from build123d import *

# Parameters (mm, degrees)
F1_DEPTH = 25.4
F2_T     = -2.54


with BuildPart() as f1:
    # F0 (on Front) → F1 (new body)
    with BuildSketch(Plane.XZ):
        with BuildLine():
            ThreePointArc((-49.597935, -5.970298), (-42.262804, 19.828677), (-16.245349, 26.3466))
            ThreePointArc((-16.245349, 26.3466), (-60.981474, 39.147241), (-49.597935, -5.970298))
        make_face()
        with BuildLine():
            ThreePointArc((-49.597935, -5.970298), (-26.099746, -1.543581), (-15.451481, 19.866116))
            ThreePointArc((-15.451481, 19.866116), (-15.650687, 23.13058), (-16.245349, 26.3466))
            ThreePointArc((-16.245349, 26.3466), (-42.262804, 19.828677), (-49.597935, -5.970298))
        make_face()
    extrude(amount=F1_DEPTH)

    # F2
    f2_openings = [f1.faces().sort_by_distance(p)[0] for p in [
        (-42.299081, -25.4, 19.866116),
    ]]
    offset(amount=F2_T, openings=f2_openings)


solid = f1.part
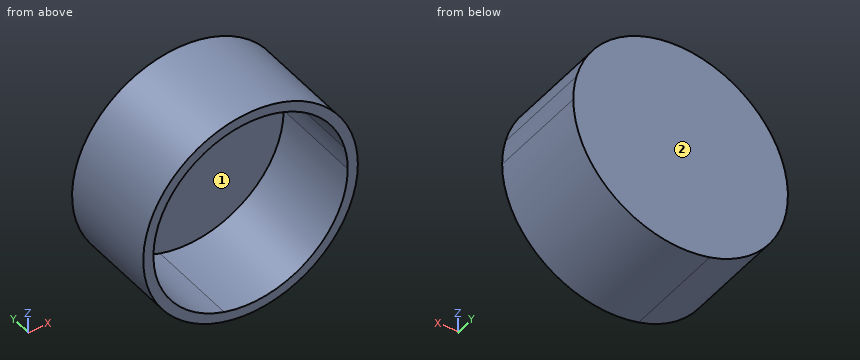
Could you check a few things on this model? Use its own coordinates, in mm. Face numbers are marked on the shaded views. Round coordinates to 2 decimals unless told otherwise and drop trailing zeros. Loops run counter-clockwise (first coordinate to the right, second up) from the corner with the lowest first, then second, coordinate; pieces in that order, holes last. Notation, with made-up numbers: (85.25, 86.5) -> (103.25, 86.5) arc R14 cw to (103.25, 109.5) -> close; hole circle Ø1 at (46, -10). An arc over 180 degrees is marked (long way). Use CSV: the item, a comma, the result in double quotes.
(1) If we mould it in two halves opening along X, with no side actions, what happens to the marked faces 1 and 2? For each: +X half, -X half, draft (parallel to the pull), parting line (faces both ways), or undercut.
Return value:
face 1,"undercut"
face 2,"draft"
(2) Suppose I cut it at C-C on z = 3. Write out the boundary of the cut face in (x, y), plus the area to 3 significant figures.
Return value:
outline,"(-63.19, -25.4) -> (-59.8, -25.4) -> (-59.8, -2.54) -> (-24.79, -2.54) -> (-24.79, -25.4) -> (-21.41, -25.4) -> (-21.41, 0) -> (-63.19, 0) -> close"
area,"261 mm²"
(3) Suppose I cut it at A-A on y = -19. Write out the boundary of the cut face in (x, z).
Return value:
outline,"(-16.25, 26.35) arc R26.85 ccw (long way) to (-15.45, 19.87) arc R26.85 ccw to start; hole (-18.71, 25.73) arc R24.31 ccw (long way) to (-17.99, 19.87) arc R24.31 ccw to start"
(4) If I drill on probe 1 along X at (y, z) = (-13.5, 20.5); probe 2 along Y at (x, z) = (-52.5, 29); probe 3 along Z at (x, y) = (-40, -15.75), over which ranges is the centre line in solid material (lowest first)? Write a range as [from, to].
Return value:
probe 1,"x = [-69.14, -66.6], [-18, -15.46]"
probe 2,"y = [-2.54, 0]"
probe 3,"z = [-6.88, -4.33], [44.06, 46.62]"
(5) Suppose I cut it at B-B on x = -65.5. Write out the boundary of the cut face in (y, z), plus the area to 3 significant figures.
Return value:
outline,"(-25.4, 6.36) -> (0, 6.36) -> (0, 33.38) -> (-25.4, 33.38) -> (-25.4, 27.12) -> (-2.54, 27.12) -> (-2.54, 12.62) -> (-25.4, 12.62) -> close"
area,"355 mm²"
(6) Will these pins go through, and if not, where does the flat tip stop? pin 1 Ø1.5 at (x, z) = (-39.5, 14) entering from -Y; pin 2 Ø4 at (x, y) = (-29, -9) entering from +Z; pin 3 Ø4 at (x, z) = (-58.5, 41) entering from +Y; pin 4 Ø4 at (x, y) = (-36.5, -6.5) entering from -Z.
Return value:
pin 1,"stops at y = -2.54"
pin 2,"stops at z = 44.22"
pin 3,"stops at y = 0"
pin 4,"stops at z = -6.71"
